from build123d import *

# Parameters (mm, degrees)
P_IDAT_VYSUNUT_M1_DEPTH                           = 9
SKICA2_R                                          = 2
SKICA2_R_2                                        = 2.55
ODEBRAT_VYSUNUT_M1_DEPTH                          = 10
SKICA4_OUTSIDE_W                                  = 50.44
SKICA4_OUTSIDE_H                                  = 20.44
ODEBRAT_VYSUNUT_M5_DEPTH                          = 4.5
KU_ELOV_ZAHLOUBEN_PRO_M4_ROUBU_SE_Z_P_D           = 4.5
KU_ELOV_ZAHLOUBEN_PRO_M4_ROUBU_SE_Z_P_DEPTH       = 13.5
KU_ELOV_ZAHLOUBEN_PRO_M4_ROUBU_SE_Z_P_CSINK_D     = 9.4
KU_ELOV_ZAHLOUBEN_PRO_M4_ROUBU_SE_Z_P_CSINK_ANGLE = 90
KU_ELOV_ZAHLOUBEN_PRO_M4_ROUBU_SE_Z_P_TIP         = 1.351936393
SKICA14_R                                         = 3.5
SKICA14_R_2                                       = 2.5
P_IDAT_VYSUNUT_M3_DEPTH                           = 1
P_IDAT_VYSUNUT_M5_REACH                           = 38.742
SKICA15_R                                         = 2


with BuildPart() as part:
    # Skica1 → Přidat vysunutím1 (new body)
    with BuildSketch(Plane.XY):
        with BuildLine():
            Line((0, 5), (30, 5))
            ThreePointArc((30, 5), (35, 0), (30, -5))
            Line((30, -5), (0, -5))
            ThreePointArc((0, -5), (-5, 0), (0, 5))
        make_face()
    extrude(amount=P_IDAT_VYSUNUT_M1_DEPTH)

    # Skica2 → Odebrat vysunutím1 (cut)
    with BuildSketch(Plane.XY.offset(9)):
        Circle(SKICA2_R)
        with Locations((30, 0)):
            Circle(SKICA2_R_2)
    extrude(amount=-ODEBRAT_VYSUNUT_M1_DEPTH, mode=Mode.SUBTRACT)

    # Skica4 outside → Odebrat vysunutím5 (cut)
    with BuildSketch(Plane(origin=(0, 0, 0), x_dir=(-1, 0, 0), z_dir=(0, 0, -1))):
        with Locations((-15, 0)):
            Rectangle(SKICA4_OUTSIDE_W, SKICA4_OUTSIDE_H)
        with BuildLine():
            Line((0, -5), (-20, -5))
            ThreePointArc((-20, -5), (-25, 0), (-20, 5))
            Line((-20, 5), (0, 5))
            ThreePointArc((0, 5), (5, 0), (0, -5))
        make_face(mode=Mode.SUBTRACT)
    extrude(amount=-ODEBRAT_VYSUNUT_M5_DEPTH, mode=Mode.SUBTRACT)

    # Kuželové zahloubení pro M4 šroubu se zápustnou hlavou plochou1
    with Locations(Plane(origin=(0, 0, 4.5), x_dir=(-1, 0, 0), z_dir=(0, 0, -1))):
        with Locations((-30, 0)):
            CounterSinkHole(KU_ELOV_ZAHLOUBEN_PRO_M4_ROUBU_SE_Z_P_D / 2, KU_ELOV_ZAHLOUBEN_PRO_M4_ROUBU_SE_Z_P_CSINK_D / 2, depth=KU_ELOV_ZAHLOUBEN_PRO_M4_ROUBU_SE_Z_P_DEPTH, counter_sink_angle=KU_ELOV_ZAHLOUBEN_PRO_M4_ROUBU_SE_Z_P_CSINK_ANGLE)
            with Locations((0, 0, -(KU_ELOV_ZAHLOUBEN_PRO_M4_ROUBU_SE_Z_P_DEPTH + KU_ELOV_ZAHLOUBEN_PRO_M4_ROUBU_SE_Z_P_TIP / 2))):  # 118° drill point
                Cone(0, KU_ELOV_ZAHLOUBEN_PRO_M4_ROUBU_SE_Z_P_D / 2, KU_ELOV_ZAHLOUBEN_PRO_M4_ROUBU_SE_Z_P_TIP, mode=Mode.SUBTRACT)

    # Skica14 → Přidat vysunutím3 (add)
    with BuildSketch(Plane.XY.offset(9)):
        with Locations((30, 0)):
            Circle(SKICA14_R)
        with Locations((30, 0)):
            Circle(SKICA14_R_2, mode=Mode.SUBTRACT)
    extrude(amount=P_IDAT_VYSUNUT_M3_DEPTH)

    # Přidat vysunutím5: up to this face of the body (flat: up to its plane)
    p_idat_vysunut_m5_end = Plane(part.part.faces().sort_by_distance((13.81286954, 0, 9))[0])
    # Skica15 → Přidat vysunutím5 (add, up to the picked face)
    with BuildSketch(Plane(origin=(0, 0, 0), x_dir=(-1, 0, 0), z_dir=(0, 0, -1)), mode=Mode.PRIVATE) as p_idat_vysunut_m5_sk1:
        with BuildLine():
            Line((-25, 0), (-5.295627791, 0))
            Line((-5.295627791, 0), (-5.295627791, -5))
            Line((-5.295627791, -5), (0, -5))
            ThreePointArc((0, -5), (5, 0), (0, 5))
            Line((0, 5), (-20, 5))
            ThreePointArc((-20, 5), (-23.535533906, 3.535533906), (-25, 0))
        make_face()
        with Locations(Location((0, 0, 0), (0, 0, 180))):
            Circle(SKICA15_R, mode=Mode.SUBTRACT)
    p_idat_vysunut_m5_tool1 = split(extrude(p_idat_vysunut_m5_sk1.sketch, amount=-P_IDAT_VYSUNUT_M5_REACH, mode=Mode.PRIVATE), bisect_by=p_idat_vysunut_m5_end, keep=Keep.BOTH, mode=Mode.PRIVATE)
    # Skica15 → Přidat vysunutím5 (add, up to the picked face)
    with BuildSketch(Plane(origin=(0, 0, 0), x_dir=(-1, 0, 0), z_dir=(0, 0, -1)), mode=Mode.PRIVATE) as p_idat_vysunut_m5_sk2:
        with BuildLine():
            Line((-7.295627791, -7), (-5.295627791, -5))
            Line((-5.295627791, -5), (-20, -5))
            ThreePointArc((-20, -5), (-21.913417162, -4.619397663), (-23.535533906, -3.535533906))
            Line((-23.535533906, -3.535533906), (-20.071067812, -7))
            Line((-20.071067812, -7), (-7.295627791, -7))
        make_face()
    p_idat_vysunut_m5_tool2 = split(extrude(p_idat_vysunut_m5_sk2.sketch, amount=-P_IDAT_VYSUNUT_M5_REACH, mode=Mode.PRIVATE), bisect_by=p_idat_vysunut_m5_end, keep=Keep.BOTH, mode=Mode.PRIVATE)
    add(p_idat_vysunut_m5_tool1.solids().sort_by(Axis((8.223408, 1.304685, 0), (0, 0, 1)))[0])
    add(p_idat_vysunut_m5_tool2.solids().sort_by(Axis((13.831058, -5.932433, 0), (0, 0, 1)))[0])


solid = part.part
Can you work these out from the model? Positions are in its coordinate system, mm. A direction names the side the tool comes from. Coordinates: 2 decimals unless noted, no trailing zeros. Order: outer loops, then holes, each group sorted by start corner. A loop starts at its lowest first (then second) coordinate and runs counter-clockwise, first axis right, second up. Notation, with made-up numbers: M 56.25,63.25 L 102.25,63.25 A10 cw 102.25,79.25 Z; hole C 41.5,-28 d7. An arc over 180 degrees is marked long. Write item = value, one per line.
(1) For pin 1 Ø1.6 at (x, z) = (2, 6.5) entering from -Y; pin 2 Ø3 at (y, z) = (-3.5, 8.5) entering from +X; pin 3 Ø5 at (y, z) = (3, 2.5) entering from -X, each with a flat end and sliding along its axis, tell me the tip position at first contact or that it passes through.
Results are:
pin_1 = -5
pin_2 = 34.58
pin_3 = -4.97
(2) I need wall thicknesses on line 1 along Y through (x, z) = (30, 8.55); line 2 along Y through (x, z) = (0, 6.5); line 3 along X through (y, z) = (-0.25, 7.25). Which ranges of each line are inside material? Lowest first, please. Write a range as [from, to].
Results are:
line_1 = [-5, -2.55], [2.55, 5]
line_2 = [-5, -2], [2, 5]
line_3 = [-4.99, -1.98], [1.98, 27.46], [32.54, 34.99]
(3) Suppose I cut it at C-C on z = 0.5. Please give me the cut outline in (x, y), plus the area to 3 significant figures.
Results are:
outline = M 0,-5 L 5.3,-5 L 7.3,-7 L 20.07,-7 L 23.54,-3.54 A5 ccw 20,5 L 0,5 A5 ccw Z; hole C 0,0 d4
area = 296 mm2
(4) For faces 5 (the face through (33.34, 1.05, 9.49)), 6 (the face through (25, 2, 4.5)), 7 (the face through (27.452, 0.112, 7.841)), which set-ups out of +Z, -Z, +X, -X, +Y, -Y let a thin tool reach every point of the face, with its end or its side?
Results are:
face_5 = +Z
face_6 = -Z, +X
face_7 = -Z
(5) Suppose I cut it at B-B on z = 7.75. Please give me the cut outline in (x, y), plus the area to 3 significant figures.
Results are:
outline = M 0,-5 L 5.3,-5 L 7.3,-7 L 20.07,-7 L 22.07,-5 L 30,-5 A5 ccw 30,5 L 0,5 A5 ccw Z; hole C 0,0 d4; hole C 30,0 d5.1
area = 375 mm2
(6) Suppose I cut it at A-A on y = 0. Please give me the cut outline in (x, z), plus the area to 3 significant figures.
Results are:
outline = M -5,0 L -2,0 L -2,9 L -5,9 Z; M 2,0 L 25,0 L 25,4.5 L 25.3,4.5 L 27.45,6.65 L 27.45,9 L 27.5,9 L 27.5,10 L 26.5,10 L 26.5,9 L 2,9 Z; M 32.5,9 L 32.55,9 L 32.55,6.65 L 34.7,4.5 L 35,4.5 L 35,9 L 33.5,9 L 33.5,10 L 32.5,10 Z
area = 253 mm2
(7) If we mould it in two halves opening along X, with no side actions, what happens to faces 1 (the face through (27.5, 0.1, 9.5)), 2 (the face through (24.65, 1.84, 2.22)), 3 (the face through (0, -2, 5)), 4 (the face through (11, -1, 9))? For each: pulls with the +X half, pulls with the -X half, needs draft (parallel to the pull), parting line crosses it, or undercut.
Results are:
face_1 = undercut
face_2 = pulls with the +X half
face_3 = undercut
face_4 = needs draft
(8) Suppose I cut it at D-D on x = 8. Please give me the cut outline in (y, z).
Results are:
outline = M -7,0 L 5,0 L 5,9 L -7,9 Z
